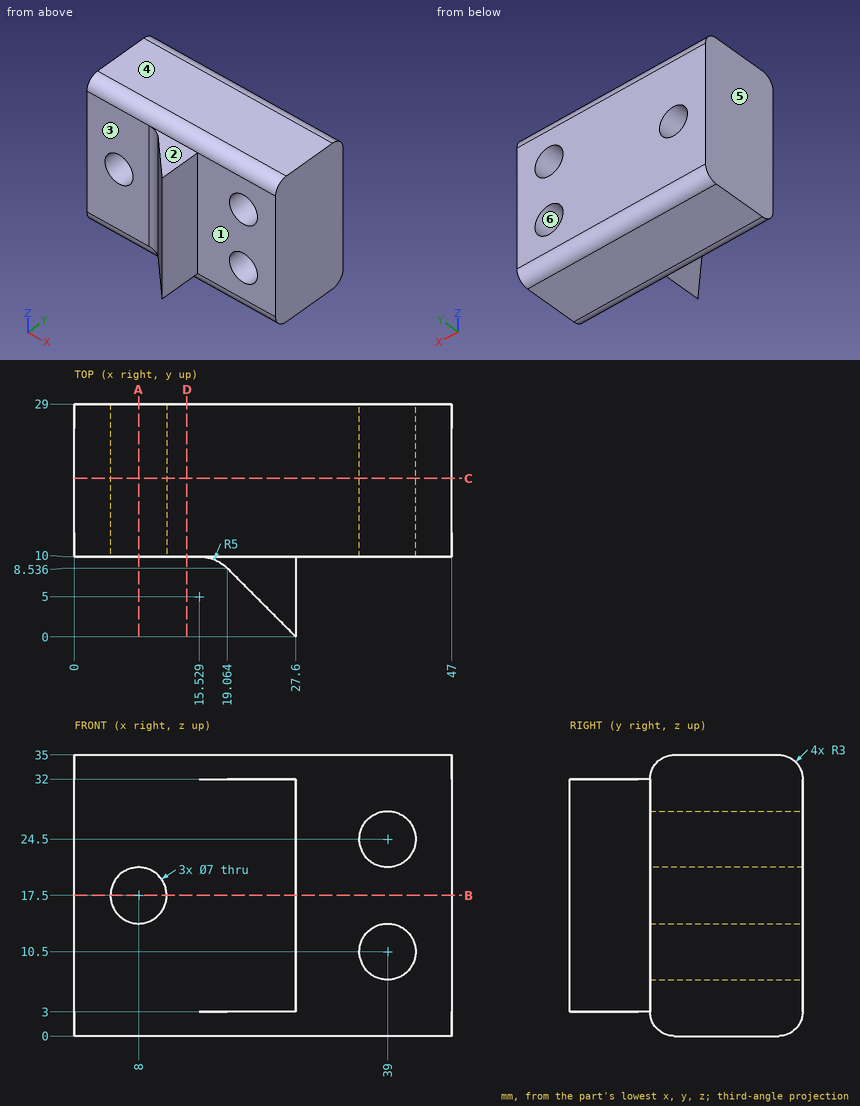
Source: three-view drawing plus pictorial views. Frame: mm from the lowest corner of the part. A direction names the side the tool comes from. Coordinates: 2 decimals unless noted, no trailing zeros. Order: outer loops, then holes, each group sorted by start corner. A loop starts at its lowest first (then second) coordinate and runs counter-clockwise, first axis right, second up. Notation, with made-up numbers: (-36.5, -34) -> (5.5, -34) arc R7 cw to (5.5, -22) -> close; hole circle Ø9 at (28.5, 87.25). An arc over 180 degrees is marked (long way). Write item = value, one per line.
(1) Pin query (flat end, axial travel): pin 1 Ø17 at (x, z) = (8, 24.5) entering from -Y (1 decimal); pin 2 Ø5 at (x, y) = (23.5, 6.5) entering from -Z; pin 3 Ø8 at (x, z) = (39, 10.5) entering from -Y. Return the tip coordinate at first contact, or that it passes through.
Solved:
pin_1 = 9.9
pin_2 = 3
pin_3 = 10
(2) Line query: line 1 (Z direction, x = 39, y = 24.5); line 2 (X direction, y = 24, z = 10.5); line 3 (Z direction, x = 8, y = 15.75). Output: solid intervals per line, ascending.
Solved:
line_1 = 0 to 7, 14 to 21, 28 to 35
line_2 = 0 to 35.5, 42.5 to 47
line_3 = 0 to 14, 21 to 35
(3) Pull-direction query (X, two-part tool) for the marked faces 4, 5 and 6; classes: pulls with the +X half, pulls with the -X half, needs draft (parallel to the pull), parting line crosses it, or undercut.
Solved:
face_4 = needs draft
face_5 = pulls with the -X half
face_6 = undercut
(4) Cut plane D-D on x = 14. Return loops of the section in (y, z).
Solved:
outline = (10, 3) arc R3 ccw to (13, 0) -> (26, 0) arc R3 ccw to (29, 3) -> (29, 32) arc R3 ccw to (26, 35) -> (13, 35) arc R3 ccw to (10, 32) -> close
(5) Cut plane C-C on y = 19.75. Return loops of the section in (x, z).
Solved:
outline = (0, 0) -> (47, 0) -> (47, 35) -> (0, 35) -> close; hole circle Ø7 at (8, 17.5); hole circle Ø7 at (39, 10.5); hole circle Ø7 at (39, 24.5)
(6) Cut plane B-B on z = 17.5. Return loops of the section in (x, y) (1 decimal).
Solved:
outline = (0, 10) -> (4.5, 10) -> (4.5, 29) -> (0, 29) -> close; (11.5, 10) -> (15.5, 10) arc R5 cw to (19.1, 8.5) -> (27.6, 0) -> (27.6, 10) -> (47, 10) -> (47, 29) -> (11.5, 29) -> close
(7) Access query for the marked faces 1, 2 and 3. Directions: +Z, -Z, +X, -X, +Y, -Y. A direction counts if a zero-diameter tool reaches every point of the face in a straight line with its end or side. Return the directions, or none.
Solved:
face_1 = +Z, -Z, +X, -Y
face_2 = +Z, +X, -X, -Y
face_3 = +Z, -Z, -X, -Y
(8) Cut plane A-A on x = 8. Return loops of the section in (y, z), plus the area to 3 significant figures.
Solved:
outline = (10, 3) arc R3 ccw to (13, 0) -> (26, 0) arc R3 ccw to (29, 3) -> (29, 14) -> (10, 14) -> close; (10, 21) -> (29, 21) -> (29, 32) arc R3 ccw to (26, 35) -> (13, 35) arc R3 ccw to (10, 32) -> close
area = 524 mm²
